Input: part model. Units: mm. Frame: model coordinates. A direction names the side the tool comes from. Round coordinates to 2 decimals unless told otherwise and drop trailing zeros. Loops run counter-clockwise (first coordinate to the right, second up) from the corner with the lowest first, then second, coordinate; pieces in that order, holes last. Notation, with made-up numbers: (-34, 80.5) -> (12, 80.5) arc R14 cw to (12, 100.5) -> close; hole circle Ø1 at (21, 63.5). An arc over 180 degrees is marked (long way). Answer as a JSON object with one key per item and string values.
```python
from build123d import *

# Parameters (mm, degrees)
SKETCH1_W           = 21.8
SKETCH1_H           = 23.2
BOSS_EXTRUDE1_DEPTH = 5.5
BOSS_EXTRUDE2_START = -5.5
SKETCH2_W           = 31.8
SKETCH2_H           = 11
BOSS_EXTRUDE2_DEPTH = 2
SKETCH3_R           = 1
CUT_EXTRUDE1_DEPTH  = 25.420278459


with BuildPart() as part:
    # Sketch1 → Boss-Extrude1 (new, symmetric)
    with BuildSketch(Plane.XY):
        Rectangle(SKETCH1_W, SKETCH1_H)
    extrude(amount=BOSS_EXTRUDE1_DEPTH, both=True)

    # Sketch2 → Boss-Extrude2 (add)
    with BuildSketch(Plane(origin=(0, 11.6, 0), x_dir=(1, 0, 0), z_dir=(0, 1, 0)).offset(BOSS_EXTRUDE2_START)):
        Rectangle(SKETCH2_W, SKETCH2_H)
    extrude(amount=-BOSS_EXTRUDE2_DEPTH)

    # Sketch3 → Cut-Extrude1 (cut, through all)
    with BuildSketch(Plane(origin=(0, 6.1, 0), x_dir=(1, 0, 0), z_dir=(0, 1, 0))):
        with Locations(Location((-13.9, 0, 0), (0, 0, 180))):
            Circle(SKETCH3_R)
        with Locations(Location((-12.9, 3, 0), (0, 0, 180))):
            Circle(SKETCH3_R)
        with Locations(Location((-12.9, -3, 0), (0, 0, 180))):
            Circle(SKETCH3_R)
        with Locations(Location((12.9, -3, 0), (0, 0, 180))):
            Circle(SKETCH3_R)
        with Locations(Location((12.9, 3, 0), (0, 0, 180))):
            Circle(SKETCH3_R)
        with Locations(Location((13.9, 0, 0), (0, 0, 180))):
            Circle(SKETCH3_R)
    extrude(amount=-CUT_EXTRUDE1_DEPTH, mode=Mode.SUBTRACT)


solid = part.part
```
1) Section A-A, the plane x = 13.5. Output: boundary loops of the cut face in (y, z), plus the area to 3 significant figures.
Output:
{"outline": "(4.1, -5.5) -> (6.1, -5.5) -> (6.1, -3.8) -> (4.1, -3.8) -> close; (4.1, -2.2) -> (6.1, -2.2) -> (6.1, -0.92) -> (4.1, -0.92) -> close; (4.1, 0.92) -> (6.1, 0.92) -> (6.1, 2.2) -> (4.1, 2.2) -> close; (4.1, 3.8) -> (6.1, 3.8) -> (6.1, 5.5) -> (4.1, 5.5) -> close", "area": "11.9 mm^2"}
2) Section D-D, the plane y = -2. Output: boundary loops of the cut face in (x, z), plus the area to 3 significant figures.
Output:
{"outline": "(-10.9, -5.5) -> (10.9, -5.5) -> (10.9, 5.5) -> (-10.9, 5.5) -> close", "area": "240 mm^2"}
3) Reachability of faces 1 (the face through (12, 4.1, 0)), 2 (the face through (-10.9, -4, 0)), 3 (the face through (10.9, 9, 0)) from +Z, -Z, +X, -X, +Y, -Y: full face, straight path, thin tool, end or side. Return the list, or none.
Output:
{"face 1": "+Z, -Z, +X, -Y", "face 2": "+Z, -Z, -X, -Y", "face 3": "+Z, -Z, +X, +Y"}
4) Section B-B, the plane z = -0.5. Output: boundary loops of the cut face in (x, y).
Output:
{"outline": "(-15.9, 4.1) -> (-14.77, 4.1) -> (-14.77, 6.1) -> (-15.9, 6.1) -> close; (-13.03, 4.1) -> (-10.9, 4.1) -> (-10.9, -11.6) -> (10.9, -11.6) -> (10.9, 4.1) -> (13.03, 4.1) -> (13.03, 6.1) -> (10.9, 6.1) -> (10.9, 11.6) -> (-10.9, 11.6) -> (-10.9, 6.1) -> (-13.03, 6.1) -> close; (14.77, 4.1) -> (15.9, 4.1) -> (15.9, 6.1) -> (14.77, 6.1) -> close"}
5) Ray query, probe 1 along X at (y, z) = (1.5, 4.75); probe 2 along Y at (x, z) = (14, -2.25). Return the intervals inside material, ascending.
Output:
{"probe 1": "x = -10.9 to 10.9", "probe 2": "y = 4.1 to 6.1"}
6) Section C-C, the plane z = -4.5. Output: boundary loops of the cut face in (x, y).
Output:
{"outline": "(-15.9, 4.1) -> (-10.9, 4.1) -> (-10.9, -11.6) -> (10.9, -11.6) -> (10.9, 4.1) -> (15.9, 4.1) -> (15.9, 6.1) -> (10.9, 6.1) -> (10.9, 11.6) -> (-10.9, 11.6) -> (-10.9, 6.1) -> (-15.9, 6.1) -> close"}
7) Draft query along Y for faces 4 (the face through (-12, 6.1, 0)), 5 (the face through (0, -11.6, 0)), 6 (the face through (0, 0, -5.5)). Return one class per face: +Y half, -Y half, draft (parallel to the pull), parting line (faces both ways), or undercut.
Output:
{"face 4": "+Y half", "face 5": "-Y half", "face 6": "draft"}
8) Contact query for flat-ended pins moving along their axis: P1, Ø1.5, axis at y = 4, z = -3, coming from the +X side; P2, Ø4, axis at x = 13.5, z = 0.5, coming from the -Y side; P3, Ø1, axis at y = -9, z = 2, coming from the -X side; P4, Ø1.8, axis at x = -13.9, z = 0, coming from the -Y side. Output: stop coordinate, or through.
Output:
{"P1": "stops at x = 15.9", "P2": "stops at y = 4.1", "P3": "stops at x = -10.9", "P4": "passes through"}
